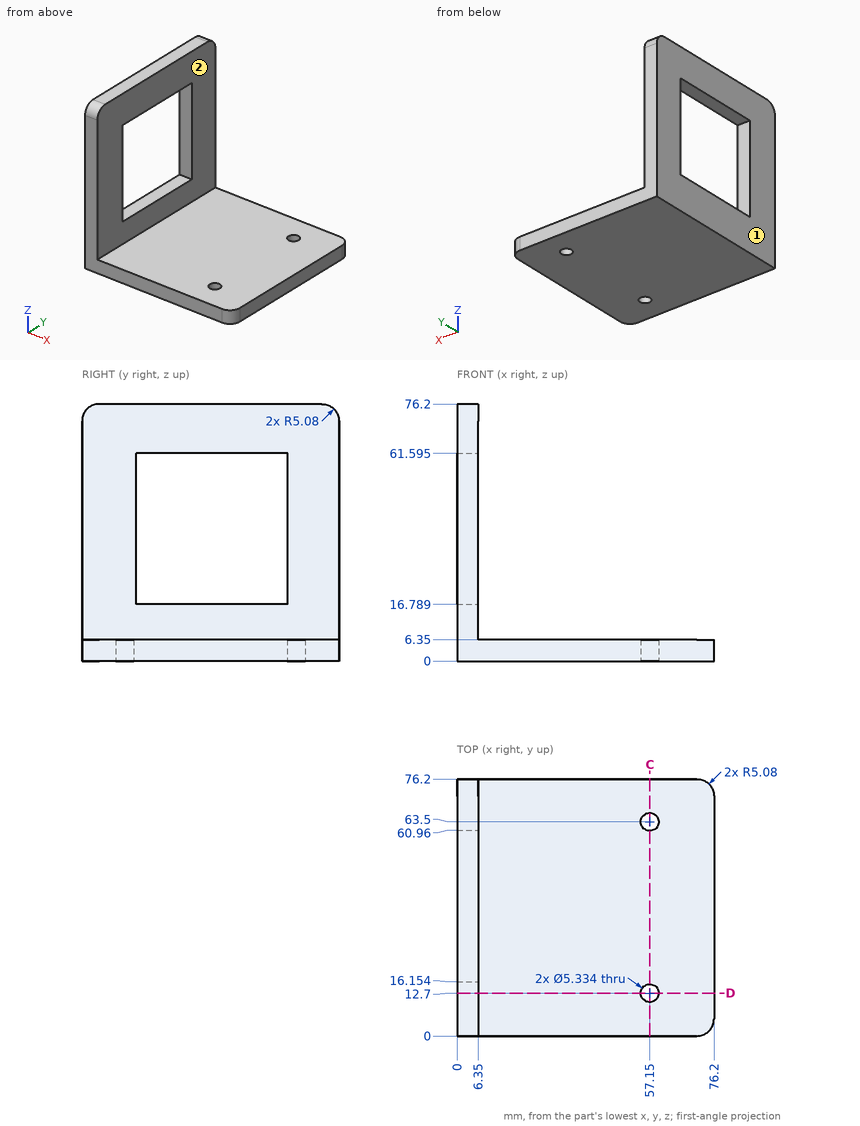
Input: dimensioned drawing with shaded views. Units: mm. Origin: part minimum x, y, z. A direction names the side the tool comes from. Coordinates: 2 decimals unless noted, no trailing zeros. Loops run counter-clockwise (first coordinate to the right, second up) from the corner with the lowest first, then second, coordinate; pieces in that order, holes last. Notation, with made-up numbers: M -38.75,59 L 19.25,59 A19 ccw 19.25,81 Z; hole C 29.25,-11.75 d11. An arc over 180 degrees is marked long. Put each result on its own line as item: value.
(1) Material intervals for probe 1 along Y at (x, z) = (57.15, 4.5); probe 2 along X at (y, z) = (61, 46); probe 3 along X at (y, z) = (63, 3), sorted ascending.
Answer sheet:
probe 1: y = 0 to 10.03, 15.37 to 60.83, 66.17 to 76.2
probe 2: x = 0 to 6.35
probe 3: x = 0 to 54.53, 59.77 to 76.2
(2) Access query for the marked faces 1 and 2. Directions: +Z, -Z, +X, -X, +Y, -Y. A direction counts if a zero-diameter tool reaches every point of the face in a straight line with its end or side. Return the directions, or none.
Answer sheet:
face 1: +Z, -Z, -X, +Y, -Y
face 2: +Z, +X, +Y, -Y
(3) First-contact query: pin 1 (6 mm diameter, centred on y = 55, z = 17.5, fed in from +X); pin 2 (21 mm diameter, centred on x = 44, y = 26.5, fed in from +Z). Flat tips, straight axial feed; report the tip coordinate or a pass-through.
Answer sheet:
pin 1: stops at x = 6.35
pin 2: stops at z = 6.35
(4) Cut plane C-C on x = 57.15. Return the cut outline in (y, z).
Answer sheet:
outline: M 0,0 L 10.03,0 L 10.03,6.35 L 0,6.35 Z; M 15.37,0 L 60.83,0 L 60.83,6.35 L 15.37,6.35 Z; M 66.17,0 L 76.2,0 L 76.2,6.35 L 66.17,6.35 Z
(5) Cut plane D-D on y = 12.7. Return the cut outline in (x, z).
Answer sheet:
outline: M 0,0 L 54.48,0 L 54.48,6.35 L 6.35,6.35 L 6.35,76.2 L 0,76.2 Z; M 59.82,0 L 76.2,0 L 76.2,6.35 L 59.82,6.35 Z
